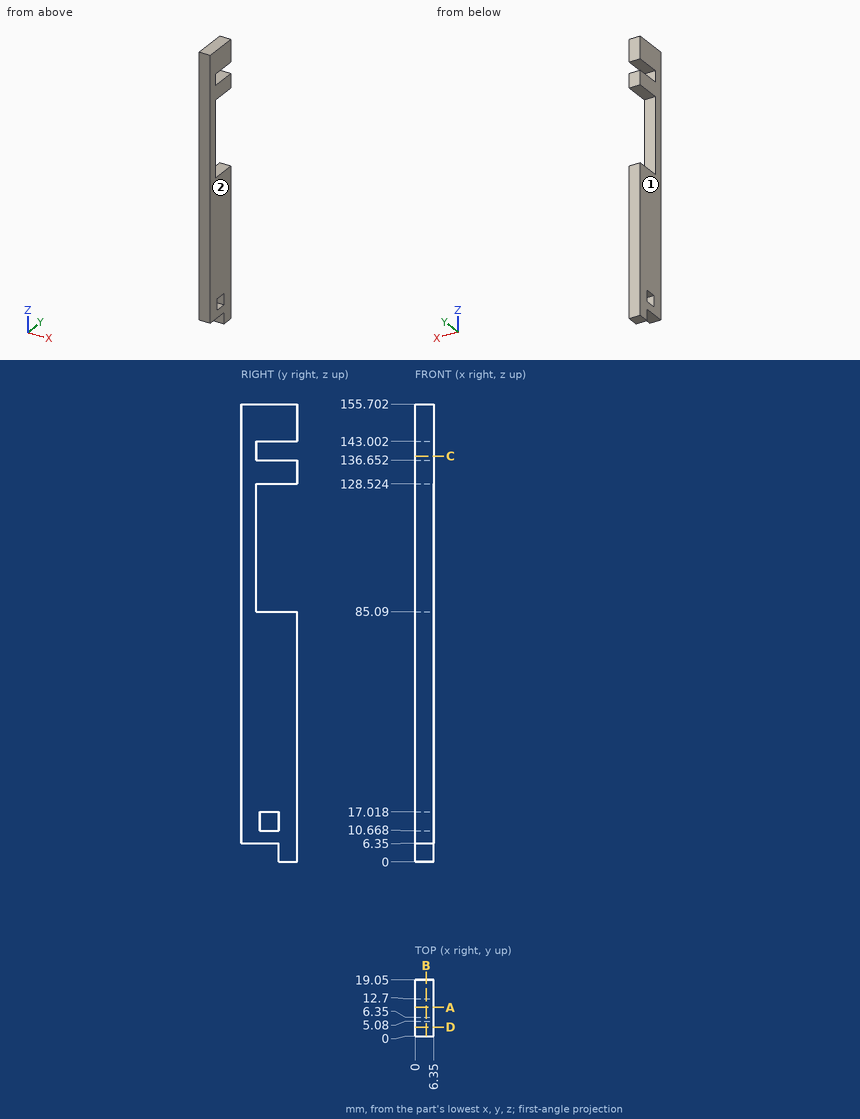
Geometry: see drawing. Coordinates: mm, zero at the bounding-box minimum. Give positions to 0.01 mm unless a question says otherwise; leave off trailing zeros. Loops run counter-clockwise (first coordinate to the right, second up) from the corner with the lowest first, then second, coordinate; pieces in that order, holes last. Notation, with made-up numbers: (4, -14.5) -> (37, -14.5) arc R35 ccw to (37, 20.5) -> close; hole circle Ø1 at (83, 88.5). An arc over 180 degrees is marked (long way). Put each result on its own line as item: value.
1. Cut plane A-A (y = 9.75). Return the cut outline in (x, z).
Taken from the geometry:
outline: (0, 6.35) -> (6.35, 6.35) -> (6.35, 10.67) -> (0, 10.67) -> close; (0, 17.02) -> (6.35, 17.02) -> (6.35, 85.09) -> (0, 85.09) -> close; (0, 128.52) -> (6.35, 128.52) -> (6.35, 136.65) -> (0, 136.65) -> close; (0, 143) -> (6.35, 143) -> (6.35, 155.7) -> (0, 155.7) -> close
2. Cut plane B-B (x = 3.75). Return the cut outline in (y, z), plus the area to 3 significant figures.
Taken from the geometry:
outline: (0, 6.35) -> (12.7, 6.35) -> (12.7, 0) -> (19.05, 0) -> (19.05, 85.09) -> (5.08, 85.09) -> (5.08, 128.52) -> (19.05, 128.52) -> (19.05, 136.65) -> (5.08, 136.65) -> (5.08, 143) -> (19.05, 143) -> (19.05, 155.7) -> (0, 155.7) -> close; hole (6.35, 10.67) -> (12.7, 10.67) -> (12.7, 17.02) -> (6.35, 17.02) -> close
area: 2,150 mm2
3. Pull-direction query (X, two-part tool) for the marked faces 1 and 2; classes: released by +X, released by -X, zero draft, split by the parting line, or undercut.
Taken from the geometry:
face 1: released by -X
face 2: released by +X
4. Pin query (flat end, axial travel): P1, Ø3, axis at x = 3.5, z = 139, coming from the +Y side; P2, Ø1.9, axis at x = 2, y = 8.5, coming from the -Z side. Return the tip coordinate at first contact, or that it passes through.
Taken from the geometry:
P1: stops at y = 5.08
P2: stops at z = 6.35
5. Cut plane D-D (y = 3). Return the cut outline in (x, z), plus the area to 3 significant figures.
Taken from the geometry:
outline: (0, 6.35) -> (6.35, 6.35) -> (6.35, 155.7) -> (0, 155.7) -> close
area: 948 mm2
6. Cut plane C-C (z = 138). Return the cut outline in (x, y).
Taken from the geometry:
outline: (0, 0) -> (6.35, 0) -> (6.35, 5.08) -> (0, 5.08) -> close
7. Ray query, line 1 along Z through (x, y) = (2.75, 6.25); line 2 along Z through (x, y) = (1.5, 12.5); line 3 along Z through (x, y) = (6, 17.5). Return the intervals inside material, ascending. Write a range as [from, to].
Taken from the geometry:
line 1: z = [6.35, 85.09], [128.52, 136.65], [143, 155.7]
line 2: z = [6.35, 10.67], [17.02, 85.09], [128.52, 136.65], [143, 155.7]
line 3: z = [0, 85.09], [128.52, 136.65], [143, 155.7]
